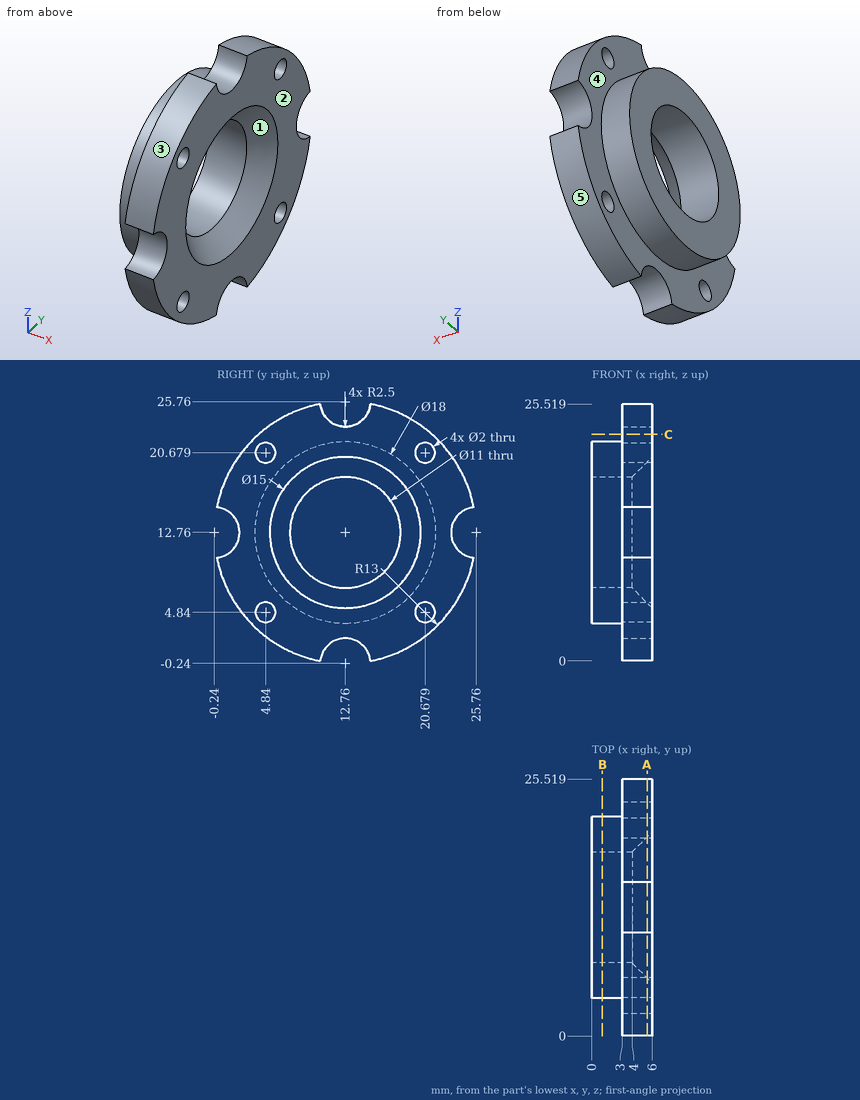
Drawing for the job (mm, zero at the part's lowest x, y, z). A direction names the side the tool comes from. Round coordinates to 2 decimals unless told otherwise and drop trailing zeros. Loops run counter-clockwise (first coordinate to the right, second up) from the corner with the lowest first, then second, coordinate; pieces in that order, holes last.
1. Wall check: probe 1 along Z at (x, y) = (4.6, 5.75) (1 decimal); probe 2 along X at (y, z) = (8, 22); probe 3 along Y at (x, z) = (0.8, 16.5) (1 decimal). Give the ranges that are in metal, low to high.
Check values:
probe 1: z = 1.8 to 4.4, 5.3 to 20.3, 21.1 to 23.7
probe 2: x = 3 to 6
probe 3: y = 4.6 to 8.7, 16.8 to 20.9
2. Band-saw the part on B-B, the plane x = 1.05. List the corners of the cut face in (y, z).
Check values:
outline: circle Ø18 at (12.76, 12.76); hole circle Ø11 at (12.76, 12.76)
3. Band-saw the part on A-A, the plane x = 5.5. List the corners of the cut face in (y, z), and give its area (3 significant figures).
Check values:
outline: (0, 10.27) arc R13 ccw to (10.27, 0) arc R2.5 cw to (15.25, 0) arc R13 ccw to (25.52, 10.27) arc R2.5 cw to (25.52, 15.25) arc R13 ccw to (15.25, 25.52) arc R2.5 cw to (10.27, 25.52) arc R13 ccw to (0, 15.25) arc R2.5 cw to start; hole circle Ø2 at (4.84, 4.84); hole circle Ø2 at (4.84, 20.68); hole circle Ø14 at (12.76, 12.76); hole circle Ø2 at (20.68, 4.84); hole circle Ø2 at (20.68, 20.68)
area: 327 mm2
4. Drop flat-ended pins along their axis: P1, Ø7.5, axis at y = 18, z = 15.5, coming from the -X side; P2, Ø12.5, axis at y = 12.76, z = 12.76, coming from the +X side; P3, Ø1.5, axis at y = 17.5, z = 4, coming from the -X side. Give the stop position or say it passes through.
Check values:
P1: stops at x = 0
P2: stops at x = 4.75
P3: stops at x = 3
5. Band-saw the part on C-C, the plane z = 22.5. List the corners of the cut face in (x, y).
Check values:
outline: (3, 4.15) - (6, 4.15) - (6, 21.37) - (3, 21.37) - close
6. Tool access for the marked faces 4 and 5: list every direction of +Z, -Z, +X, -X, +Y, -Y with a clear straight run to the whole face (end or side of a thin tool).
Check values:
face 4: -X
face 5: -Z, +X, -X, +Y
7. Mould opens along Z. For the marked faces 1, 2 and 3 say: +Z half, -Z half, draft (parallel to the pull), parting line (faces both ways), or undercut.
Check values:
face 1: undercut
face 2: draft
face 3: +Z half
